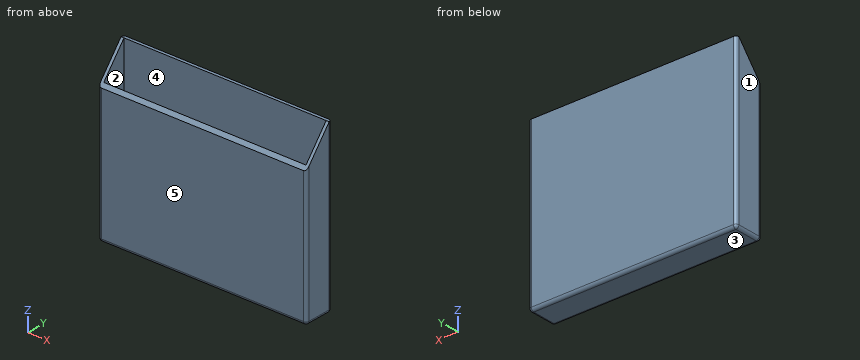
```python
from build123d import *

# Parameters (mm, degrees)
F0_W     = 140
F0_H     = 20
F1_DEPTH = 2
F2_W     = 140
F2_H     = 20
F2_W_2   = 136
F2_H_2   = 16
F3_DEPTH = 110
F5_DEPTH = 160
F6_R     = 2


with BuildPart() as f1:
    # F0 (on Top) → F1 (new body)
    with BuildSketch(Plane.XY):
        Rectangle(F0_W, F0_H)
    extrude(amount=F1_DEPTH)

    # F2 (on face) → F3 (join)
    with BuildSketch(Plane.XY.offset(2)):
        Rectangle(F2_W, F2_H)
        Rectangle(F2_W_2, F2_H_2, mode=Mode.SUBTRACT)
    extrude(amount=F3_DEPTH)

    # F4 (on face) → F5 (cut)
    with BuildSketch(Plane(origin=(-70, 0, 0), x_dir=(0, -1, 0), z_dir=(-1, 0, 0))):
        Polygon((10, 112), (-8, 112), (10, 90.232462), align=None)
    extrude(amount=-F5_DEPTH, mode=Mode.SUBTRACT)

    # F6
    f6_edges = [f1.edges().sort_by_distance(p)[0] for p in [
        (-70, -10, 45.116231),
        (70, -10, 45.116231),
        (-70, 10, 56),
        (70, 10, 56),
        (0, -10, 0),
        (70, 0, 0),
        (0, 10, 0),
        (-70, 0, 0),
    ]]
    fillet(f6_edges, radius=F6_R)


solid = f1.part
```
Can you work these out from the model? Positions are in its coordinate system, mm. Face numbers are marked on the shaded views. A direction names the side the tool comes from. Coordinates: 2 decimals unless noted, no trailing zeros. Loops run counter-clockwise (first coordinate to the right, second up) from the corner with the lowest first, then second, coordinate; pieces in that order, holes last. Notation, with made-up numbers: (83.5, -29.75) -> (104.5, -29.75) arc R17 cw to (104.5, -10.75) -> close; hole circle Ø3 at (12.5, -16). An arc over 180 degrees is marked (long way). Put each result on its own line as item: value. Start each with the question number.
Q1. If I drill on line 1 (X direction, y = -4.5, z = 46.5); line 2 (Y direction, x = -54, z = 61); line 3 (Z direction, x = 18.5, y = 7.75), over which ranges is the centre line in solid material (lowest first)? Write a range as [from, to].
Q2. I want a section at C-C (y = -2.5). Write out the boundary of the cut face in (x, z).
Q3. I want a section at B-B (x = 53). Write out the boundary of the cut face in (y, z).
Q4. I'm going to push flat-ended pins straight in: P1, Ø1, axis at x = -53, z = 95.5, coming from the -Y side; P2, Ø2, axis at x = -39.5, y = 4, coming from the +Z side. Where does each tip first touch, or does it pass through?
Q5. I want a section at A-A (z = 27). Write out the boundary of the cut face in (x, y).
Q6. Thinking about a two-plate mould opening in X: for the marked faces 1, 2 and 3, which applies, pulls with the +X half, pulls with the -X half, needs draft (parallel to the pull), parting line crosses it, or undercut?
Q7. For the marked faces 4 and 5, which set-ups out of +Z, -Z, +X, -X, +Y, -Y let a thin tool reach every point of the face, with its end or its side?
Taken from the geometry:
1. line 1: x = [-70, -68], [68, 70]
1. line 2: y = [-10, -8], [8, 10]
1. line 3: z = [0, 2]
2. outline: (-70, 2) arc R2 ccw to (-68, 0) -> (68, 0) arc R2 ccw to (70, 2) -> (70, 99.3) -> (68, 99.3) -> (68, 2) -> (-68, 2) -> (-68, 99.3) -> (-70, 99.3) -> close
3. outline: (-10, 2) arc R2 ccw to (-8, 0) -> (8, 0) arc R2 ccw to (10, 2) -> (10, 112) -> (8, 112) -> (8, 2) -> (-8, 2) -> (-8, 92.65) -> (-10, 90.23) -> close
4. P1: stops at y = 8
4. P2: stops at z = 2
5. outline: (-70, -8) arc R2 ccw to (-68, -10) -> (68, -10) arc R2 ccw to (70, -8) -> (70, 8) arc R2 ccw to (68, 10) -> (-68, 10) arc R2 ccw to (-70, 8) -> close; hole (-68, -8) -> (68, -8) -> (68, 8) -> (-68, 8) -> close
6. face 1: pulls with the -X half
6. face 2: undercut
6. face 3: needs draft
7. face 4: +Z
7. face 5: +Z, -Z, +X, -X, -Y
